Design review of the part built by this model. Coordinates are the model's own, in mm. Face numbers are marked on the shaded views. A direction names the side the tool comes from. Coordinates: 2 decimals unless noted, no trailing zeros. Write each loop counter-clockwise with the first axis right and the second up, starting at its lowest first coordinate (ties: lowest second). Pieces come first, ordered by that corner, then holes. Notation, with made-up numbers: (-34.5, -21) - (21.5, -21) arc R13 ccw to (21.5, -13) - close; hole circle Ø1 at (5, 26). An arc over 180 degrees is marked (long way). One line per item, written item: value.
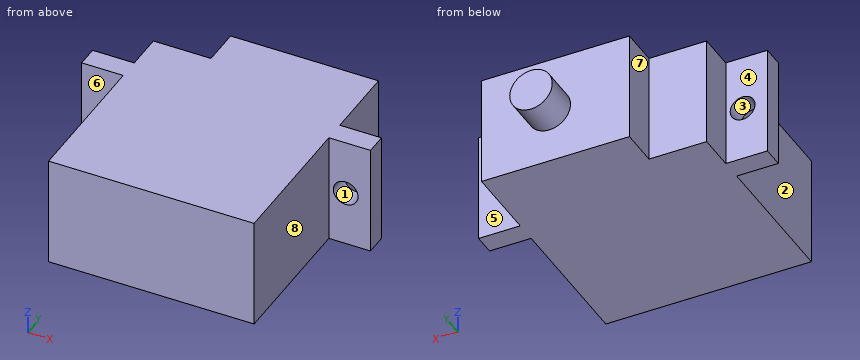
from build123d import *

# Parameters (mm, degrees)
BOSS_EXTRUDE1_DEPTH = 12.5
SKETCH2_R           = 1.4
CUT_EXTRUDE1_DEPTH  = 12.5
SKETCH3_R           = 2.4
BOSS_EXTRUDE2_DEPTH = 4


with BuildPart() as part:
    # Sketch1 → Boss-Extrude1 (new body)
    with BuildSketch(Plane.XY):
        Polygon((0, 18.8), (0, 23), (6.504024825, 23), (6.504024825, 27.3), (23.2, 27.3), (23.2, 23), (23.2, 18.8), (27.9, 18.8), (27.9, 16.4), (23.2, 16.4), (23.2, 0), (0, 0), (0, 16.4), (-4.7, 16.4), (-4.7, 18.8), align=None)
    extrude(amount=BOSS_EXTRUDE1_DEPTH)

    # Sketch2 → Cut-Extrude1 (cut)
    with BuildSketch(Plane(origin=(0, 27.3, 0), x_dir=(1, 0, 0), z_dir=(0, 1, 0))):
        with Locations(Location((-1.9, -6.25, 0), (0, 0, 270))):
            Circle(SKETCH2_R)
        with Locations(Location((25.1, -6.25, 0), (0, 0, 270))):
            Circle(SKETCH2_R)
    extrude(amount=-CUT_EXTRUDE1_DEPTH, mode=Mode.SUBTRACT)

    # Sketch3 → Boss-Extrude2 (add)
    with BuildSketch(Plane(origin=(0, 27.3, 0), x_dir=(1, 0, 0), z_dir=(0, 1, 0))):
        with Locations(Location((15.556949647, -6.25, 0), (0, 0, 270))):
            Circle(SKETCH3_R)
    extrude(amount=BOSS_EXTRUDE2_DEPTH)


solid = part.part
1. Consider section A-A, the plane x = -1.9. Write out the cut boundary in (y, z), then the cut area to 3 significant figures.
Answer block:
outline: (16.4, 0) - (18.8, 0) - (18.8, 4.85) - (16.4, 4.85) - close; (16.4, 7.65) - (18.8, 7.65) - (18.8, 12.5) - (16.4, 12.5) - close
area: 23.3 mm^2
2. Consider section B-B, the plane z = 6.25. Write out the cut boundary in (x, y), then the cut area to 3 significant figures.
Answer block:
outline: (-4.7, 16.4) - (-3.3, 16.4) - (-3.3, 18.8) - (-4.7, 18.8) - close; (-0.5, 16.4) - (0, 16.4) - (0, 0) - (23.2, 0) - (23.2, 16.4) - (23.7, 16.4) - (23.7, 18.8) - (23.2, 18.8) - (23.2, 27.3) - (17.96, 27.3) - (17.96, 31.3) - (13.16, 31.3) - (13.16, 27.3) - (6.5, 27.3) - (6.5, 23) - (0, 23) - (0, 18.8) - (-0.5, 18.8) - close; (26.5, 16.4) - (27.9, 16.4) - (27.9, 18.8) - (26.5, 18.8) - close
area: 634 mm^2
3. Consider section D-D, the plane x = 7.5. Write out the cut boundary in (y, z).
Answer block:
outline: (0, 0) - (27.3, 0) - (27.3, 12.5) - (0, 12.5) - close
4. Wall thickness on line 1 along X through (y, z) = (18, 6.25); line 2 along Y through (x, z) = (3.5, 3); line 3 along X through (y, z) = (21, 3.5): over which ranges is each line inside the solid? List them lowest first.
Answer block:
line 1: x = -4.7 to -3.3, -0.5 to 23.7, 26.5 to 27.9
line 2: y = 0 to 23
line 3: x = 0 to 23.2
5. For the marked faces 5, 6, 7 and 8, list the 3-axis set-ups (+Z, -Z, +X, -X, +Y, -Y) from which the entire face can be reached by the end or side of a thin tool; tool diameter is ignored.
Answer block:
face 5: +Z, -Z, +X, +Y
face 6: +Z, -Z, -X, -Y
face 7: +Z, -Z, -X, +Y
face 8: +Z, -Z, +X, -Y
6. Mouldability with a two-part tool opening along X and no side actions: class the marked faces 1, 2, 3 and 4 as released by +X, released by -X, zero draft, split by the parting line, or undercut.
Answer block:
face 1: undercut
face 2: released by -X
face 3: undercut
face 4: zero draft
7. Consider section C-C, the plane z = 9.5. Write out the cut boundary in (x, y), then the cut area to 3 significant figures.
Answer block:
outline: (-4.7, 16.4) - (0, 16.4) - (0, 0) - (23.2, 0) - (23.2, 16.4) - (27.9, 16.4) - (27.9, 18.8) - (23.2, 18.8) - (23.2, 27.3) - (6.5, 27.3) - (6.5, 23) - (0, 23) - (0, 18.8) - (-4.7, 18.8) - close
area: 628 mm^2
8. Insertion check: pin 1 Ø6 at (y, z) = (5, 6.5) entering from -X; pin 2 Ø5 at (x, z) = (3, 5.5) entering from +Y; pin 3 Ø1.4 at (x, z) = (26, 6.5) entering from +Y. Each pin has a flat end and moves straight along its axis. Give the tip position at first contact, or say it passes through.
Answer block:
pin 1: stops at x = 0
pin 2: stops at y = 23
pin 3: stops at y = 18.8
